from build123d import *

# Parameters (mm, degrees)
SKETCH_R   = 3
SKETCH_R_2 = 3.75
PAD_DEPTH  = 12


with BuildPart() as part:
    # Sketch → Pad (new body)
    with BuildSketch(Plane.XY):
        with BuildLine():
            Line((-43, -10), (43, -10))
            ThreePointArc((43, -10), (44.414214, -9.414214), (45, -8))
            Line((45, -8), (45, 10))
            ThreePointArc((45, 10), (44.694859, 11.061816), (43.872547, 11.799628))
            Line((10.872547, 27.799628), (43.872547, 11.799628))
            ThreePointArc((10.872547, 27.799628), (10.447629, 27.949264), (10, 28))
            Line((-10, 28), (10, 28))
            ThreePointArc((-10, 28), (-10.447629, 27.949264), (-10.872547, 27.799628))
            Line((-43.872547, 11.799628), (-10.872547, 27.799628))
            ThreePointArc((-43.872547, 11.799628), (-44.694859, 11.061816), (-45, 10))
            Line((-45, -8), (-45, 10))
            ThreePointArc((-45, -8), (-44.414214, -9.414214), (-43, -10))
        make_face()
        with Locations((-35, 0)):
            Circle(SKETCH_R, mode=Mode.SUBTRACT)
        with Locations((35, 0)):
            Circle(SKETCH_R, mode=Mode.SUBTRACT)
        with Locations((0, 20)):
            Circle(SKETCH_R_2, mode=Mode.SUBTRACT)
    extrude(amount=PAD_DEPTH)


solid = part.part
Part model, mm, in its own coordinate system. Coordinates: 2 decimals unless noted, no trailing zeros. Order: outer loops, then holes, each group sorted by start corner. A loop starts at its lowest first (then second) coordinate and runs counter-clockwise, first axis right, second up. Notation, with made-up numbers: (52, 84.25) - (109, 84.25) arc R7 cw to (109, 88.25) - close; hole circle Ø4 at (30, -26). An arc over 180 degrees is marked (long way). Use CSV: the item, a comma, the result in double quotes.
Item 1: Mould opens along X. For faces 1 (the face through (-45, 1, 6)), 2 (the face through (-1, -10, 6)), 3 (the face through (-38, 0, 6)) say: +X half, -X half, draft (parallel to the pull), parting line (faces both ways), or undercut.
Solved:
face 1,"-X half"
face 2,"draft"
face 3,"undercut"
Item 2: Probe probe 1 along Y at (x, z) = (-36, 1.25); probe 2 along X at (y, z) = (1.5, 7.5); probe 3 along Y at (x, z) = (-1.5, 9.5). List the from-to ranges inside material, lowest first.
Solved:
probe 1,"y = -10 to -2.83, 2.83 to 15.62"
probe 2,"x = -45 to -37.6, -32.4 to 32.4, 37.6 to 45"
probe 3,"y = -10 to 16.56, 23.44 to 28"
Item 3: Saw through at C-C on x = 0. Give the cut face in (y, z), and give its area (3 significant figures).
Solved:
outline,"(-10, 0) - (16.25, 0) - (16.25, 12) - (-10, 12) - close; (23.75, 0) - (28, 0) - (28, 12) - (23.75, 12) - close"
area,"366 mm²"
Item 4: Drop a flat-ended pin along its axis: P1, Ø7, axis at x = 35, y = 0, coming from the -Z side. Give the stop position or say it passes through.
Solved:
P1,"stops at z = 0"
Item 5: Saw through at A-A on y = 0. Give the cut face in (x, z), and give its area (3 significant figures).
Solved:
outline,"(-45, 0) - (-38, 0) - (-38, 12) - (-45, 12) - close; (-32, 0) - (32, 0) - (32, 12) - (-32, 12) - close; (38, 0) - (45, 0) - (45, 12) - (38, 12) - close"
area,"936 mm²"
Item 6: Saw through at B-B on z = 7. Give the cut face in (x, y).
Solved:
outline,"(-45, -8) arc R2 ccw to (-43, -10) - (43, -10) arc R2 ccw to (45, -8) - (45, 10) arc R2 ccw to (43.87, 11.8) - (10.87, 27.8) arc R2 ccw to (10, 28) - (-10, 28) arc R2 ccw to (-10.87, 27.8) - (-43.87, 11.8) arc R2 ccw to (-45, 10) - close; hole circle Ø6 at (-35, 0); hole circle Ø7.5 at (0, 20); hole circle Ø6 at (35, 0)"
Item 7: Saw through at D-D on x = 35. Give the cut face in (y, z), and give its area (3 significant figures).
Solved:
outline,"(-10, 0) - (-3, 0) - (-3, 12) - (-10, 12) - close; (3, 0) - (16.1, 0) - (16.1, 12) - (3, 12) - close"
area,"241 mm²"
